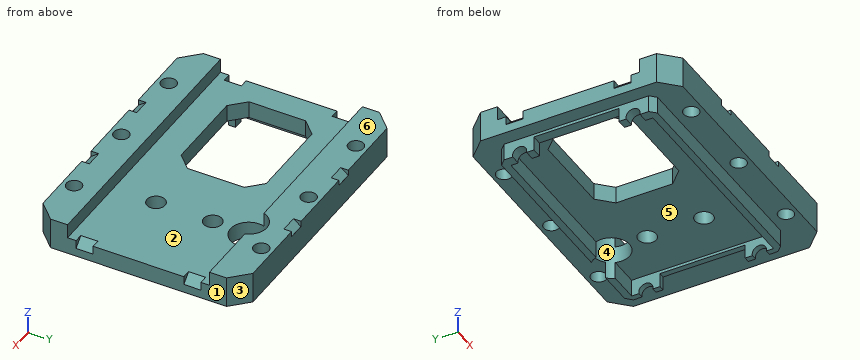
```python
from build123d import *
from OCP.BRepFilletAPI import BRepFilletAPI_MakeChamfer

# Parameters (mm, degrees)
SKETCH_1_W                  = 48.5
SKETCH_1_H                  = 37
EXTRUDE_1_DEPTH             = 7.5
SKETCH_2_W                  = 4.5
SKETCH_2_H                  = 25
CUT_EXTRUDE_1_DEPTH         = 54.398977368
SKETCH_3_W                  = 41
SKETCH_3_H                  = 27.5
EXTRUDE_2_DEPTH             = 3.028
SKETCH_4_W                  = 38.25
SKETCH_4_H                  = 25
CUT_EXTRUDE_2_DEPTH         = 3.028
CUT_EXTRUDE_3_DEPTH         = 49.015109955
CUT_EXTRUDE_4_DEPTH         = 52.139033859
CUT_EXTRUDE_5_DEPTH         = 32.090983966
HOLE_WIZARD_2_5_2_5_1_D     = 2.5
HOLE_WIZARD_2_5_2_5_1_DEPTH = 1.75
HOLE_WIZARD_2_5_2_5_2_D     = 2.5
HOLE_WIZARD_2_5_2_5_2_DEPTH = 6
HOLE_WIZARD_2_5_2_5_3_D     = 2.5
HOLE_WIZARD_2_5_2_5_3_DEPTH = 4.25
HOLE_WIZARD_2_7_2_7_1_D     = 2.7
CHAMFER_1_SIZE              = 3
SKETCH_17_W                 = 3
SKETCH_17_H                 = 4
CUT_EXTRUDE_8_DEPTH         = 3
CHAMFER_2_SIZE              = 3
CHAMFER_2_SIZE_2            = 3.981134465
SKETCH_19_W                 = 2
SKETCH_19_H                 = 3
CUT_EXTRUDE_9_DEPTH         = 1.5
CHAMFER_3_SIZE              = 2
CHAMFER_4_SIZE              = 1
SKETCH_20_R                 = 3.2
CUT_EXTRUDE_10_DEPTH        = 21.5
SKETCH_21_W                 = 19.5
SKETCH_21_H                 = 15
CUT_EXTRUDE_11_DEPTH        = 21.5
CHAMFER_5_SIZE              = 2.5
SKETCH_22_W                 = 9
SKETCH_22_H                 = 15
CUT_EXTRUDE_12_DEPTH        = 51.5
SKETCH_23_W                 = 48.5
SKETCH_23_H                 = 2
CUT_EXTRUDE_13_DEPTH        = 50
SKETCH_24_R                 = 1.6
CUT_EXTRUDE_14_DEPTH        = 10


# Some blends are built 0.0001 mm under size
with BuildPart() as part:
    # 草图1 → 凸台-拉伸1 (new body)
    with BuildSketch(Plane(origin=(0, 0, 5.028), x_dir=(-1, 0, 0), z_dir=(0, 0, -1))):
        Rectangle(SKETCH_1_W, SKETCH_1_H)
    extrude(amount=-EXTRUDE_1_DEPTH)

    # 草图2 → 切除-拉伸1 (cut, through all)
    with BuildSketch(Plane(origin=(24.25, 0, 0), x_dir=(0, 0, -1), z_dir=(1, 0, 0))):
        with Locations((-10.278, 0)):
            Rectangle(SKETCH_2_W, SKETCH_2_H)
    extrude(amount=-CUT_EXTRUDE_1_DEPTH, mode=Mode.SUBTRACT)

    # 草图3 → 凸台-拉伸2 (add)
    with BuildSketch(Plane(origin=(0, 0, 5.028), x_dir=(-1, 0, 0), z_dir=(0, 0, -1))):
        with Locations((1.25, 0)):
            Rectangle(SKETCH_3_W, SKETCH_3_H)
    extrude(amount=EXTRUDE_2_DEPTH)

    # 草图4 → 切除-拉伸2 (cut)
    with BuildSketch(Plane(origin=(0, 0, 2), x_dir=(-1, 0, 0), z_dir=(0, 0, -1))):
        with Locations((0.875, 0)):
            Rectangle(SKETCH_4_W, SKETCH_4_H)
    extrude(amount=-CUT_EXTRUDE_2_DEPTH, mode=Mode.SUBTRACT)

    # 草图5 → 切除-拉伸3 (cut, through all)
    with BuildSketch(Plane.ZY.offset(-18.25)):
        with BuildLine():
            Line((2, 7.034395212), (2, -7.034395212))
            ThreePointArc((2, -7.034395212), (4.278, 0), (2, 7.034395212))
        make_face()
    extrude(amount=-CUT_EXTRUDE_3_DEPTH, mode=Mode.SUBTRACT)

    # 草图6 → 切除-拉伸4 (cut, through all)
    with BuildSketch(Plane.ZY.offset(21.75)):
        with BuildLine():
            Line((2, 7.034395212), (2, -7.034395212))
            ThreePointArc((2, -7.034395212), (4.278, 0), (2, 7.034395212))
        make_face()
    extrude(amount=-CUT_EXTRUDE_4_DEPTH, mode=Mode.SUBTRACT)

    # 草图7 → 切除-拉伸5 (cut, through all)
    with BuildSketch(Plane.XY.offset(8.028)):
        with BuildLine():
            Line((-7.978419869, 7.029222073), (-13.021580131, 7.029222073))
            ThreePointArc((-13.021580131, 7.029222073), (-17.801221513, 4.934335949), (-19.5, 0))
            ThreePointArc((-19.5, 0), (-17.801221513, -4.934335949), (-13.021580131, -7.029222073))
            Line((-13.021580131, -7.029222073), (-7.978419869, -7.029222073))
            ThreePointArc((-7.978419869, -7.029222073), (-3.198778487, -4.934335949), (-1.5, 0))
            ThreePointArc((-1.5, 0), (-3.198778487, 4.934335949), (-7.978419869, 7.029222073))
        make_face()
    extrude(amount=-CUT_EXTRUDE_5_DEPTH, mode=Mode.SUBTRACT)

    # Ø2.5 (2.5) 直径孔1
    with Locations(Plane.ZY.offset(21.75)):
        with Locations((2.278, 10)):
            Hole(HOLE_WIZARD_2_5_2_5_1_D / 2, depth=HOLE_WIZARD_2_5_2_5_1_DEPTH)

    # Ø2.5 (2.5) 直径孔2
    with Locations(Plane.ZY.offset(-18.25)):
        with Locations((2.278, -10), (2.278, 10)):
            Hole(HOLE_WIZARD_2_5_2_5_2_D / 2, depth=HOLE_WIZARD_2_5_2_5_2_DEPTH)

    # Ø2.5 (2.5) 直径孔3
    with Locations(Plane(origin=(-20, 0, 0), x_dir=(0, 0, -1), z_dir=(1, 0, 0))):
        with Locations((-2.278, -10)):
            Hole(HOLE_WIZARD_2_5_2_5_3_D / 2, depth=HOLE_WIZARD_2_5_2_5_3_DEPTH)

    # Ø2.7 (2.7) 直径孔1 (through all)
    with Locations(Plane.XY.offset(12.528)):
        with Locations((0, -16.5), (-15, -16.5), (15, -16.5), (0, 16.5), (-15, 16.5), (15, 16.5)):
            Hole(HOLE_WIZARD_2_7_2_7_1_D / 2)

    # 倒角1
    chamfer_1_edges = [part.edges().sort_by_distance(p)[0] for p in [
        (-24.25, 18.5, 8.778),
        (-24.25, -18.5, 8.778),
        (24.25, -18.5, 8.778),
        (24.25, 18.5, 8.778),
    ]]
    chamfer(chamfer_1_edges, length=CHAMFER_1_SIZE)

    # 草图17 → 切除-拉伸8 (cut)
    with BuildSketch(Plane.XY.offset(12.528)):
        with Locations((-7.5, -16.5)):
            Rectangle(SKETCH_17_W, SKETCH_17_H)
        with Locations((7.5, -16.5)):
            Rectangle(SKETCH_17_W, SKETCH_17_H)
        with Locations((7.5, 16.5)):
            Rectangle(SKETCH_17_W, SKETCH_17_H)
        with Locations((-7.5, 16.5)):
            Rectangle(SKETCH_17_W, SKETCH_17_H)
    extrude(amount=-CUT_EXTRUDE_8_DEPTH, mode=Mode.SUBTRACT)

    # 倒角2
    chamfer_2_edges_1 = [part.edges().sort_by_distance(p)[0] for p in [
        (7.5, -14.5, 9.528),
    ]]
    chamfer_2_side_1 = [part.faces().sort_by_distance(p)[0] for p in [
        (7.5, -14.5, 9.588),
    ]]
    chamfer_2_edges_2 = [part.edges().sort_by_distance(p)[0] for p in [
        (-7.5, -14.5, 9.528),
    ]]
    chamfer_2_side_2 = [part.faces().sort_by_distance(p)[0] for p in [
        (-7.5, -14.5, 9.588),
    ]]
    chamfer_2_edges_3 = [part.edges().sort_by_distance(p)[0] for p in [
        (-7.5, 14.5, 9.528),
    ]]
    chamfer_2_side_3 = [part.faces().sort_by_distance(p)[0] for p in [
        (-7.5, 14.5, 9.588),
    ]]
    chamfer_2_edges_4 = [part.edges().sort_by_distance(p)[0] for p in [
        (7.5, 14.5, 9.528),
    ]]
    chamfer_2_side_4 = [part.faces().sort_by_distance(p)[0] for p in [
        (7.5, 14.5, 9.588),
    ]]
    chamfer_2 = BRepFilletAPI_MakeChamfer(part.part.solid().wrapped)
    for e in chamfer_2_edges_1:
        chamfer_2.Add(CHAMFER_2_SIZE - 0.0001, CHAMFER_2_SIZE_2 - 0.0001, e.wrapped, chamfer_2_side_1[0].wrapped)
    for e in chamfer_2_edges_2:
        chamfer_2.Add(CHAMFER_2_SIZE - 0.0001, CHAMFER_2_SIZE_2 - 0.0001, e.wrapped, chamfer_2_side_2[0].wrapped)
    for e in chamfer_2_edges_3:
        chamfer_2.Add(CHAMFER_2_SIZE - 0.0001, CHAMFER_2_SIZE_2 - 0.0001, e.wrapped, chamfer_2_side_3[0].wrapped)
    for e in chamfer_2_edges_4:
        chamfer_2.Add(CHAMFER_2_SIZE - 0.0001, CHAMFER_2_SIZE_2 - 0.0001, e.wrapped, chamfer_2_side_4[0].wrapped)
    add(Compound.cast(chamfer_2.Shape()), mode=Mode.REPLACE)  # a hair under: the kernel refuses the full size

    # 草图19 → 切除-拉伸9 (cut)
    with BuildSketch(Plane.XY.offset(8.028)):
        with Locations((-23.25, -9.5)):
            Rectangle(SKETCH_19_W, SKETCH_19_H)
        with Locations((-23.25, 9.5)):
            Rectangle(SKETCH_19_W, SKETCH_19_H)
        with Locations((23.25, 9.5)):
            Rectangle(SKETCH_19_W, SKETCH_19_H)
        with Locations((23.25, -9.5)):
            Rectangle(SKETCH_19_W, SKETCH_19_H)
    extrude(amount=-CUT_EXTRUDE_9_DEPTH, mode=Mode.SUBTRACT)

    # 倒角3
    # the kernel refuses this chamfer: 2 mm, written as the material it adds along each edge
    with BuildSketch(Plane(origin=(22.25, 11, 6.528), x_dir=(0.9996219169112968, 0, -0.02749587661058651), z_dir=(0, -1, 0))) as chamfer_3_piece_1_section:
        Polygon((CHAMFER_3_SIZE * 0.999621916911, CHAMFER_3_SIZE * 0.0274958766106), (-CHAMFER_3_SIZE * 0.0274958766106, CHAMFER_3_SIZE * 0.999621916911), (0, 0), align=None)
    chamfer_3_piece_1 = extrude(amount=8.143365976, mode=Mode.PRIVATE)
    chamfer_3_piece_1 = split(chamfer_3_piece_1, bisect_by=Plane(origin=(22.95, 9.5, 8.028), z_dir=(0, 0, -1)), keep=Keep.TOP, mode=Mode.PRIVATE)
    add(chamfer_3_piece_1)
    with BuildSketch(Plane(origin=(22.25, -11, 6.528), x_dir=(0.9996219169112968, 0, -0.02749587661058651), z_dir=(0, 1, 0))) as chamfer_3_piece_2_section:
        Polygon((CHAMFER_3_SIZE * 0.999621916911, -CHAMFER_3_SIZE * 0.0274958766106), (-CHAMFER_3_SIZE * 0.0274958766106, -CHAMFER_3_SIZE * 0.999621916911), (0, 0), align=None)
    chamfer_3_piece_2 = extrude(amount=8.143365976, mode=Mode.PRIVATE)
    chamfer_3_piece_2 = split(chamfer_3_piece_2, bisect_by=Plane(origin=(22.95, -9.5, 8.028), z_dir=(0, 0, -1)), keep=Keep.TOP, mode=Mode.PRIVATE)
    add(chamfer_3_piece_2)
    with BuildSketch(Plane(origin=(-22.25, 11, 6.528), x_dir=(-0.9996219169112968, 0, -0.02749587661058651), z_dir=(0, -1, 0))) as chamfer_3_piece_3_section:
        Polygon((CHAMFER_3_SIZE * 0.999621916911, -CHAMFER_3_SIZE * 0.0274958766106), (-CHAMFER_3_SIZE * 0.0274958766106, -CHAMFER_3_SIZE * 0.999621916911), (0, 0), align=None)
    chamfer_3_piece_3 = extrude(amount=8.143365976, mode=Mode.PRIVATE)
    chamfer_3_piece_3 = split(chamfer_3_piece_3, bisect_by=Plane(origin=(-22.95, 9.5, 8.028), z_dir=(0, 0, -1)), keep=Keep.TOP, mode=Mode.PRIVATE)
    add(chamfer_3_piece_3)
    with BuildSketch(Plane(origin=(-22.25, -16.143365976, 6.528), x_dir=(-0.9996219169112968, 0, -0.02749587661058651), z_dir=(0, 1, 0))) as chamfer_3_piece_4_section:
        Polygon((CHAMFER_3_SIZE * 0.999621916911, CHAMFER_3_SIZE * 0.0274958766106), (-CHAMFER_3_SIZE * 0.0274958766106, CHAMFER_3_SIZE * 0.999621916911), (0, 0), align=None)
    chamfer_3_piece_4 = extrude(amount=13.286731952, mode=Mode.PRIVATE)
    chamfer_3_piece_4 = split(chamfer_3_piece_4, bisect_by=Plane(origin=(-22.95, -9.5, 8.028), z_dir=(0, 0, -1)), keep=Keep.TOP, mode=Mode.PRIVATE)
    chamfer_3_piece_4 = split(chamfer_3_piece_4, bisect_by=Plane(origin=(-26.6, -13.15, 7.128), z_dir=(0.7071067811865476, 0.7071067811865476, 0)), keep=Keep.TOP, mode=Mode.PRIVATE)
    add(chamfer_3_piece_4)

    # 倒角4
    chamfer_4_edges = [part.edges().sort_by_distance(p)[0] for p in [
        (-21.75, 13.75, 3.514),
        (19.25, 13.75, 3.514),
        (19.25, -13.75, 3.514),
        (-21.75, -13.75, 3.514),
    ]]
    chamfer(chamfer_4_edges, length=CHAMFER_4_SIZE)

    # 草图20 → 切除-拉伸10 (cut)
    with BuildSketch(Plane(origin=(0, 0, 2), x_dir=(-1, 0, 0), z_dir=(0, 0, -1))):
        with Locations(Location((-10, 11.5, 0), (0, 0, 18.209956864))):
            Circle(SKETCH_20_R)
    extrude(amount=-CUT_EXTRUDE_10_DEPTH, mode=Mode.SUBTRACT)

    # 草图21 → 切除-拉伸11 (cut)
    with BuildSketch(Plane.XY.offset(8.028)):
        with Locations((-10, 0)):
            Rectangle(SKETCH_21_W, SKETCH_21_H)
    extrude(amount=-CUT_EXTRUDE_11_DEPTH, mode=Mode.SUBTRACT)

    # 倒角5
    chamfer_5_edges = [part.edges().sort_by_distance(p)[0] for p in [
        (-0.25, 7.5, 6.528),
        (-0.25, -7.5, 6.528),
        (-19.75, -7.5, 6.528),
        (-19.75, 7.5, 6.528),
    ]]
    chamfer(chamfer_5_edges, length=CHAMFER_5_SIZE)

    # 草图22 → 切除-拉伸12 (cut)
    with BuildSketch(Plane(origin=(19.25, 0, 0), x_dir=(0, 0, -1), z_dir=(1, 0, 0))):
        Rectangle(SKETCH_22_W, SKETCH_22_H)
    extrude(amount=-CUT_EXTRUDE_12_DEPTH, mode=Mode.SUBTRACT)

    # 草图23 → 切除-拉伸13 (cut)
    with BuildSketch(Plane.XZ.offset(18.5)):
        with Locations((0, 11.528)):
            Rectangle(SKETCH_23_W, SKETCH_23_H)
    extrude(amount=-CUT_EXTRUDE_13_DEPTH, mode=Mode.SUBTRACT)

    # 草图24 → 切除-拉伸14 (cut)
    with BuildSketch(Plane.XY.offset(8.028)):
        with Locations((9.703840341, 5)):
            Circle(SKETCH_24_R)
        with Locations(Location((9.703840341, -5, 0), (0, 0, 180))):
            Circle(SKETCH_24_R)
    extrude(amount=-CUT_EXTRUDE_14_DEPTH, mode=Mode.SUBTRACT)


solid = part.part
```
Build history of the part. All positions in model axes, mm. Face numbers are marked on the shaded views. A direction names the side the tool comes from. Coordinates: 2 decimals unless noted, no trailing zeros. Order: outer loops, then holes, each group sorted by start corner. A loop starts at its lowest first (then second) coordinate and runs counter-clockwise, first axis right, second up. Notation, with made-up numbers: (10, 41) -> (65, 41) arc R15 cw to (65, 52) -> close; hole circle Ø7 at (26, -38). An arc over 180 degrees is marked (long way). Answer in a Markdown table with one row per item. Add a question column.
Q1. Mould opens along X. For the marked faces 3, 4, 5 and 6 say: +X half, -X half, draft (parallel to the pull), parting line (faces both ways), or undercut.
Q2. Band-saw the part on B-B, the plane y = -16.5. List the corners of the cut face in (x, z), then the cut area to 3 significant figures.
Q3. Band-saw the part on A-A, the plane x = -10. List the corners of the cut face in (y, z).
Q4. Wall check: line 1 along Y through (x, z) = (-15, 6.75); line 2 along X through (y, z) = (-5, 7.25); line 3 along Y through (x, z) = (1.5, 4.25). Give the ranges that are in metal, low to high. Write a range as [from, to].
Q5. Band-saw the part on C-C, the plane x = 15. List the corners of the cut face in (y, z).
Q6. Drop flat-ended pins along their axis: pin 1 (5 mm diameter, centred on x = 8.5, y = 1, fed in from +Z); pin 2 (1.6 mm diameter, centred on x = -15, y = 16.5, fed in from -Z); pin 3 (1.5 mm diameter, centred on y = 8.5, z = 4, fed in from -X); pin 4 (1.6 mm diameter, centred on x = -23.5, z = 7, fed in from +Y). Give the stop position or say it passes through.
Q7. Which spindle directions (+Z, -Z, +X, -X, +Y, -Y) get a long thin tool onto all of the face, cutting with end or side? Do the marked faces 1 and 2. Say none if no direction does.
Q8. Band-saw the part on D-D, the plane y = -4.5. List the corners of the cut face in (x, z), then the cut area to 3 significant figures.
Answers follow:
| question | item | result |
|---|---|---|
| 1 | face 3 | +X half |
| 1 | face 4 | undercut |
| 1 | face 5 | undercut |
| 1 | face 6 | draft |
| 2 | outline | (-23.25, 5.03) -> (-16.35, 5.03) -> (-16.35, 10.53) -> (-23.25, 10.53) -> close; (-13.65, 5.03) -> (-1.35, 5.03) -> (-1.35, 10.53) -> (-13.65, 10.53) -> close; (1.35, 5.03) -> (13.65, 5.03) -> (13.65, 10.53) -> (1.35, 10.53) -> close; (16.35, 5.03) -> (23.25, 5.03) -> (23.25, 10.53) -> (16.35, 10.53) -> close |
| 2 | area | 211 mm^2 |
| 3 | outline | (-18.5, 5.03) -> (-13.75, 5.03) -> (-13.75, 2) -> (-12.5, 2) -> (-12.5, 5.03) -> (-7.5, 5.03) -> (-7.5, 8.03) -> (-12.5, 8.03) -> (-12.5, 10.53) -> (-18.5, 10.53) -> close; (7.5, 5.03) -> (12.5, 5.03) -> (12.5, 2) -> (13.75, 2) -> (13.75, 5.03) -> (18.5, 5.03) -> (18.5, 10.53) -> (12.5, 10.53) -> (12.5, 8.03) -> (7.5, 8.03) -> close |
| 4 | line 1 | [-18.5, -17.85], [-15.15, -7.5], [7.5, 15.15], [17.85, 18.5] |
| 4 | line 2 | [-24.25, -19.75], [-0.25, 8.1], [11.3, 24.25] |
| 4 | line 3 | [-13.75, -12.5], [12.5, 13.75] |
| 5 | outline | (-18.5, 5.03) -> (-17.85, 5.03) -> (-17.85, 10.53) -> (-18.5, 10.53) -> close; (-15.15, 5.03) -> (-13.75, 5.03) -> (-13.75, 2) -> (-12.5, 2) -> (-12.5, 5.03) -> (12.5, 5.03) -> (12.5, 2) -> (13.75, 2) -> (13.75, 5.03) -> (15.15, 5.03) -> (15.15, 10.53) -> (12.5, 10.53) -> (12.5, 8.03) -> (-12.5, 8.03) -> (-12.5, 10.53) -> (-15.15, 10.53) -> close; (17.85, 5.03) -> (18.5, 5.03) -> (18.5, 10.53) -> (17.85, 10.53) -> close |
| 6 | pin 1 | z = 8.03 |
| 6 | pin 2 | through |
| 6 | pin 3 | x = -21.75 |
| 6 | pin 4 | y = 17.05 |
| 7 | face 1 | +Z, -Z, +X, +Y, -Y |
| 7 | face 2 | +Z, +X, -X |
| 8 | outline | (-24.25, 5.03) -> (-21.75, 5.03) -> (-21.75, 4.5) -> (-20, 4.5) -> (-20, 5.03) -> (-19.75, 5.03) -> (-19.75, 8.03) -> (-24.25, 8.03) -> close; (-0.25, 5.03) -> (8.18, 5.03) -> (8.18, 8.03) -> (-0.25, 8.03) -> close; (11.22, 5.03) -> (18.25, 5.03) -> (18.25, 4.5) -> (19.25, 4.5) -> (19.25, 5.03) -> (24.25, 5.03) -> (24.25, 8.03) -> (11.22, 8.03) -> close |
| 8 | area | 79.3 mm^2 |
